```python
from build123d import *


with BuildPart() as part:
    # Body: sweep along a path in PathSke
    with BuildLine(Plane.XY) as body_path:
        Line((10, 0.5), (0, 0.5))
        ThreePointArc((0, 0.5), (-0.788240781, 0.597036875), (-1.529411765, 0.882352941))
        ThreePointArc((-1.529411765, 0.882352941), (-3, 0), (-1.529411765, -0.882352941))
        ThreePointArc((-1.529411765, -0.882352941), (-0.788240781, -0.597036875), (0, -0.5))
        Line((0, -0.5), (12.5, -0.5))
    # SectionSke → Body (sweep)
    with BuildSketch(Plane(origin=(10, 0, 0), x_dir=(0, 0, -1), z_dir=(1, 0, 0))):
        with BuildLine():
            Line((-0.499996, 0.002), (0.499996, 0.002))
            ThreePointArc((0.499996, 0.002), (0, 0.5), (-0.499996, 0.002))
        make_face()
    sweep(path=body_path.line)


solid = part.part
```
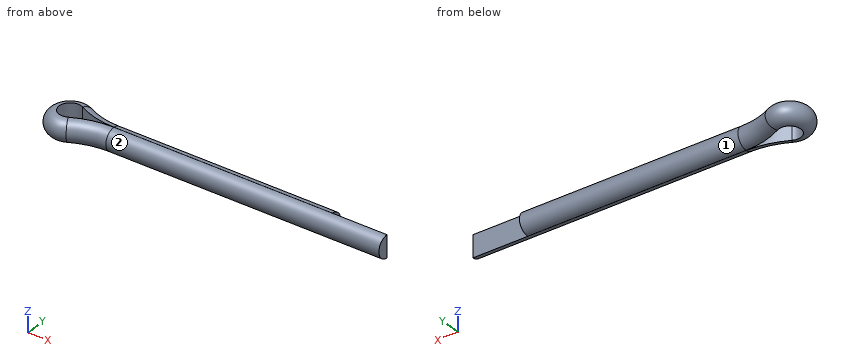
Can you work these out from the model? Positions are in its coordinate system, mm. Face numbers are marked on the shaded views. A direction names the side the tool comes from. Round coordinates to 2 decimals unless told otherwise and drop trailing zeros. Answer in a Markdown table with one row per item.
Item 1: If I drill on probe 1 along Y at (x, z) = (-2, 0); probe 2 along Y at (x, z) = (-2, 0.25); probe 3 along X at (y, z) = (-0.3, 0.3), over which ranges is the centre line in solid material (lowest first)?
Answer block:
| item | result |
|---|---|
| probe 1 | -1 to -0.5, 0.5 to 1 |
| probe 2 | -0.93 to -0.5, 0.5 to 0.93 |
| probe 3 | -2.85 to -2.4, -1.46 to 12.5 |
Item 2: Will these pins go through, and if not, where does the flat tip stop? P1, Ø0.9, axis at x = -2, y = 0, coming from the +Z side; P2, Ø0.5, axis at x = 8, z = 0, coming from the +Y side.
Answer block:
| item | result |
|---|---|
| P1 | through |
| P2 | y = 0.5 |
Item 3: On a 3-axis mill with a long thin cutter (end or side, diameter ignored), from which of +Z, -Z, +X, -X, +Y, -Y can I reach the whole of each face in a straight line? I mean the marked faces 1 and 2. Say none if no direction works.
Answer block:
| item | result |
|---|---|
| face 1 | +X, +Y |
| face 2 | +X, -Y |
